Part model, mm, in its own coordinate system. A direction names the side the tool comes from. Round coordinates to 2 decimals unless told otherwise and drop trailing zeros. Write each loop counter-clockwise with the first axis right and the second up, starting at its lowest first coordinate (ties: lowest second). Pieces come first, ordered by that corner, then holes.
```python
from build123d import *

# Parameters (mm, degrees)
SKETCH1_W                                           = 110
SKETCH1_H                                           = 42
BOSS_EXTRUDE1_DEPTH                                 = 7
F_4_4_4_4_DIAMETER_HOLE1_D                          = 4.4
CBORE_FOR_M4_HEX_SOCKET_HEAD_CAP_SCREW1_D           = 4.3
CBORE_FOR_M4_HEX_SOCKET_HEAD_CAP_SCREW1_CBORE_D     = 8
CBORE_FOR_M4_HEX_SOCKET_HEAD_CAP_SCREW1_CBORE_DEPTH = 5
SKETCH18_R                                          = 1.75
CUT_EXTRUDE1_DEPTH                                  = 10
FILLET1_R                                           = 5
CHAMFER1_SIZE                                       = 0.5
CUT_EXTRUDE2_DEPTH                                  = 2.5
FILLET2_R                                           = 1
CHAMFER2_SIZE                                       = 0.5


with BuildPart() as part:
    # Sketch1 → Boss-Extrude1 (new body)
    with BuildSketch(Plane(origin=(0, 0, 0), x_dir=(1, 0, 0), z_dir=(0, 1, 0))):
        Rectangle(SKETCH1_W, SKETCH1_H)
    extrude(amount=BOSS_EXTRUDE1_DEPTH)

    # Ø4.4 (4.4) Diameter Hole1 (through all)
    with Locations(Plane(origin=(0, 0, 0), x_dir=(-1, 0, 0), z_dir=(0, -1, 0))):
        with Locations((-40, 15), (-40, -15), (40, -15), (40, 15)):
            Hole(F_4_4_4_4_DIAMETER_HOLE1_D / 2)

    # CBORE for M4 Hex Socket Head Cap Screw1 (through all)
    with Locations(Plane(origin=(0, 0, 0), x_dir=(-1, 0, 0), z_dir=(0, -1, 0))):
        with Locations((-15, 15), (15, 15), (-15, -15), (15, -15)):
            CounterBoreHole(CBORE_FOR_M4_HEX_SOCKET_HEAD_CAP_SCREW1_D / 2, CBORE_FOR_M4_HEX_SOCKET_HEAD_CAP_SCREW1_CBORE_D / 2, CBORE_FOR_M4_HEX_SOCKET_HEAD_CAP_SCREW1_CBORE_DEPTH)

    # Sketch18 → Cut-Extrude1 (cut)
    with BuildSketch(Plane.XZ):
        with Locations(Location((50, 8.5, 0), (0, 0, 270))):
            Circle(SKETCH18_R)
        with Locations(Location((50, -8.5, 0), (0, 0, 270))):
            Circle(SKETCH18_R)
        with BuildLine():
            Line((-50, 10.2), (-45, 10.2))
            ThreePointArc((-45, 10.2), (-43.3, 8.5), (-45, 6.8))
            Line((-45, 6.8), (-50, 6.8))
            ThreePointArc((-50, 6.8), (-51.7, 8.5), (-50, 10.2))
        make_face()
        with BuildLine():
            Line((-50, -6.8), (-45, -6.8))
            ThreePointArc((-45, -6.8), (-43.3, -8.5), (-45, -10.2))
            Line((-45, -10.2), (-50, -10.2))
            ThreePointArc((-50, -10.2), (-51.7, -8.5), (-50, -6.8))
        make_face()
    extrude(amount=-CUT_EXTRUDE1_DEPTH, mode=Mode.SUBTRACT)

    # Fillet1
    fillet1_edges = [part.edges().sort_by_distance(p)[0] for p in [
        (55, 3.5, 21),
        (-55, 3.5, 21),
        (-55, 3.5, -21),
        (55, 3.5, -21),
    ]]
    fillet(fillet1_edges, radius=FILLET1_R)

    # Chamfer1
    chamfer1_edges = [part.edges().sort_by_distance(p)[0] for p in [
        (-55, 0, 0),
        (55, 0, 0),
        (0, 0, 21),
        (0, 0, -21),
        (-53.535533906, 0, 19.535533906),
        (53.535533906, 0, 19.535533906),
        (53.535533906, 0, -19.535533906),
        (-53.535533906, 0, -19.535533906),
        (-42.2, 0, -15),
        (-42.2, 0, 15),
        (37.8, 0, 15),
        (37.8, 0, -15),
        (-11, 0, 15),
        (19, 0, 15),
        (-11, 0, -15),
        (19, 0, -15),
        (-51.7, 0, -8.5),
        (-47.5, 0, -10.2),
        (-43.3, 0, -8.5),
        (-47.5, 0, -6.8),
        (50, 0, 10.25),
        (50, 0, -6.75),
        (-51.7, 0, 8.5),
        (-47.5, 0, 6.8),
        (-43.3, 0, 8.5),
        (-47.5, 0, 10.2),
    ]]
    chamfer(chamfer1_edges, length=CHAMFER1_SIZE)

    # Sketch22 → Cut-Extrude2 (cut)
    with BuildSketch(Plane(origin=(0, 7, 0), x_dir=(1, 0, 0), z_dir=(0, 1, 0))):
        Polygon((46.795706006, -8.5), (48.397853003, -11.275), (51.602146997, -11.275), (53.204293994, -8.5), (51.602146997, -5.725), (48.397853003, -5.725), align=None)
        Polygon((46.795706006, 8.5), (48.397853003, 5.725), (51.602146997, 5.725), (53.204293994, 8.5), (51.602146997, 11.275), (48.397853003, 11.275), align=None)
    extrude(amount=-CUT_EXTRUDE2_DEPTH, mode=Mode.SUBTRACT)

    # Fillet2
    fillet2_edges = [part.edges().sort_by_distance(p)[0] for p in [
        (46.795706006, 5.75, 8.5),
        (48.397853003, 5.75, 5.725),
        (51.602146997, 5.75, 5.725),
        (53.204293994, 5.75, 8.5),
        (51.602146997, 5.75, 11.275),
        (48.397853003, 5.75, 11.275),
        (46.795706006, 5.75, -8.5),
        (48.397853003, 5.75, -11.275),
        (51.602146997, 5.75, -11.275),
        (53.204293994, 5.75, -8.5),
        (51.602146997, 5.75, -5.725),
        (48.397853003, 5.75, -5.725),
    ]]
    fillet(fillet2_edges, radius=FILLET2_R)

    # Chamfer2
    chamfer2_edges = [part.edges().sort_by_distance(p)[0] for p in [
        (52.403220496, 7, 9.8875),
        (50, 7, 11.275),
        (52.403220496, 7, 7.1125),
        (50, 7, 5.725),
        (47.596779504, 7, 7.1125),
        (47.596779504, 7, 9.8875),
        (50, 7, -5.725),
        (47.596779504, 7, -7.1125),
        (47.596779504, 7, -9.8875),
        (50, 7, -11.275),
        (52.403220496, 7, -9.8875),
        (52.403220496, 7, -7.1125),
        (51.524796728, 7, 11.141025404),
        (53.049593456, 7, 8.5),
        (51.524796728, 7, 5.858974596),
        (48.475203272, 7, 5.858974596),
        (46.950406544, 7, 8.5),
        (48.475203272, 7, 11.141025404),
        (48.475203272, 7, -5.858974596),
        (46.950406544, 7, -8.5),
        (48.475203272, 7, -11.141025404),
        (51.524796728, 7, -11.141025404),
        (53.049593456, 7, -8.5),
        (51.524796728, 7, -5.858974596),
    ]]
    chamfer(chamfer2_edges, length=CHAMFER2_SIZE)


solid = part.part
```
Q1. Mould opens along X. For faces 1 (the flat face through (-17, 5, 17)), 2 (the flat face through (-1, 4, -21)), 3 (the cylindrical face through (53, 4, -20)), 4 (the cylindrical face through (-54, 4, 19)) say: +X half, -X half, draft (parallel to the pull), parting line (faces both ways), or undercut.
Values follow:
face 1: undercut
face 2: draft
face 3: +X half
face 4: -X half
Q2. Drop flat-ended pins along their axis: pin 1 (2.5 mm diameter, centred on x = -40, z = 15, fed in from +Y); pin 2 (7 mm diameter, centred on x = -15, z = 15, fed in from -Y); pin 3 (6.5 mm diameter, centred on x = 14, z = 14.5, fed in from -Y). Give the stop position or say it passes through.
Values follow:
pin 1: passes through
pin 2: stops at y = 5
pin 3: stops at y = 0.13
Q3. Wall check: L1, parallel to X at y = 6.3, z = -15; L2, parallel to X at y = 3, z = -15; L3, parallel to Z at x = -15, y = 5.9. Give the ranges that are in metal, low to high.
Values follow:
L1: x = -55 to -42.2, -37.8 to -17.15, -12.85 to 12.85, 17.15 to 37.8, 42.2 to 55
L2: x = -55 to -42.2, -37.8 to -19, -11 to 11, 19 to 37.8, 42.2 to 55
L3: z = -21 to -17.15, -12.85 to 12.85, 17.15 to 21
Q4. Which spindle directions (+Z, -Z, +X, -X, +Y, -Y) get a long thin tool onto all of the face, cutting with end or side? Do faces 5 (the flat face through (52.396, 5.514, 9.9)), 6 (the cylindrical face through (-12.05, 2.72, -17.7)), 7 (the conical face through (53.241, 0.135, -19.314)), 8 (the flat face through (-48, 4, -6.8)). Say none if no direction does.
Values follow:
face 5: +Y
face 6: -Y
face 7: -Z, +X, -Y
face 8: +Y, -Y
Q5. Cut at A-A on x = 15. Write the cut outline in (y, z).
Values follow:
outline: (0, -20.5) - (0.5, -21) - (7, -21) - (7, -17.15) - (5, -17.15) - (5, -19) - (0.5, -19) - (0, -19.5) - close; (0, -10.5) - (0.5, -11) - (5, -11) - (5, -12.85) - (7, -12.85) - (7, 12.85) - (5, 12.85) - (5, 11) - (0.5, 11) - (0, 10.5) - close; (0, 19.5) - (0.5, 19) - (5, 19) - (5, 17.15) - (7, 17.15) - (7, 21) - (0.5, 21) - (0, 20.5) - close
Q6. Cut at B-B on y = 3. State how many separate pieces and enclosed holes the cut face has, plus the area to 3 significant figures.
Values follow:
separate pieces: 1
enclosed holes: 12
area: 4,270 mm2
